The model under review builds one solid part; all positions refer to its coordinate system, in mm. A direction names the side the tool comes from. Give positions to 0.01 mm unless a question says otherwise; leave off trailing zeros. Order: outer loops, then holes, each group sorted by start corner. A loop starts at its lowest first (then second) coordinate and runs counter-clockwise, first axis right, second up. Notation, with made-up numbers: (5.5, -17) - (29.5, -17) arc R31 ccw to (29.5, 7) - close; hole circle Ø4 at (4, -2). An arc over 180 degrees is marked (long way). Use CSV: the item, a comma, the result in double quotes.
```python
from build123d import *

# Parameters (mm, degrees)
F2_DEPTH = 25


with BuildPart() as f1:
    # F0 (on Front) → F1 (revolve)
    with BuildSketch(Plane.XZ):
        Polygon((0, 40), (0, 12), (125, 12), (125, 30), (75, 25), (50, 40), align=None)
    revolve(axis=Axis((34.2099070549, 0, 0), (1, 0, 0)))

    # F2 (add): a face of the model
    f2_faces = [f1.faces().sort_by_distance(p)[0] for p in [
        (125, 0, -12.8485281374),
    ]]
    extrude(f2_faces, amount=F2_DEPTH)


solid = f1.part
```
Item 1: Mouldability with a two-part tool opening along X and no side actions: class faces 1 (the face through (0, -9.4, 8.3)), 2 (the face through (24.65, 39.05, -8.67)), 3 (the face through (150, 13, 0)), 4 (the face through (73.44, -7.79, 24.74)) as pulls with the +X half, pulls with the -X half, needs draft (parallel to the pull), parting line crosses it, or undercut.
Results list:
face 1,"pulls with the -X half"
face 2,"needs draft"
face 3,"pulls with the +X half"
face 4,"undercut"
Item 2: Take a section at C-C, the plane x = 122. Give the boundary of the cut face in (y, z).
Results list:
outline,"circle Ø59.4 at (0, 0); hole circle Ø24 at (0, 0)"
Item 3: Take a section at A-A, the plane z = 0. Give the boundary of the cut face in (x, y).
Results list:
outline,"(0, -40) - (50, -40) - (75, -25) - (125, -30) - (150, -30) - (150, -12) - (0, -12) - close; (0, 12) - (150, 12) - (150, 30) - (125, 30) - (75, 25) - (50, 40) - (0, 40) - close"
Item 4: Tool access review of faces 5 (the face through (73.95, -0.53, -11.99)), 6 (the face through (137.32, -1.32, -29.97)), 7 (the face through (99.65, -8.25, 26.197)): name each direction out of +Z, -Z, +X, -X, +Y, -Y from which nothing blocks a thin tool from reaching the whole face with its end or side.
Results list:
face 5,"+X, -X"
face 6,"+X"
face 7,"none"
Item 5: Wall thickness on L1, parallel to Z at x = 44.5, y = 0; L2, parallel to Y at x = 87, z = 0; L3, parallel to Z at x = 34.5, y = 8.5: over which ranges is each line inside the solid? List them lowest first.
Results list:
L1,"z = -40 to -12, 12 to 40"
L2,"y = -26.2 to -12, 12 to 26.2"
L3,"z = -39.09 to -8.47, 8.47 to 39.09"
Item 6: Take a section at D-D, the plane x = 32. Give the boundary of the cut face in (y, z).
Results list:
outline,"circle Ø80 at (0, 0); hole circle Ø24 at (0, 0)"
Item 7: Clearance check with flat-ended pins moving along their axes: pin 1 (2 mm diameter, centred on x = 56, z = 8, fed in from +Y); pin 2 (3 mm diameter, centred on x = 70.5, z = -21.5, fed in from +Y); pin 3 (3 mm diameter, centred on x = 86.5, y = -6.5, fed in from -Z). State where each tip first meets the part, or that it passes through.
Results list:
pin 1,"stops at y = 36.16"
pin 2,"stops at y = 19.63"
pin 3,"stops at z = -25.7"
